Here's how the part is built. I have some questions about the finished solid (model axes, mm). Face numbers are marked on the shaded views. Coordinates: 2 decimals unless noted, no trailing zeros. Write each loop counter-clockwise with the first axis right and the second up, starting at its lowest first coordinate (ties: lowest second). Pieces come first, ordered by that corner, then holes. Notation, with made-up numbers: (55.5, 11) -> (69.5, 11) arc R22 ccw to (69.5, 25) -> close; hole circle Ø7 at (61.5, 42). An arc over 180 degrees is marked (long way). Use a Markdown table: item, result. Add a question column.
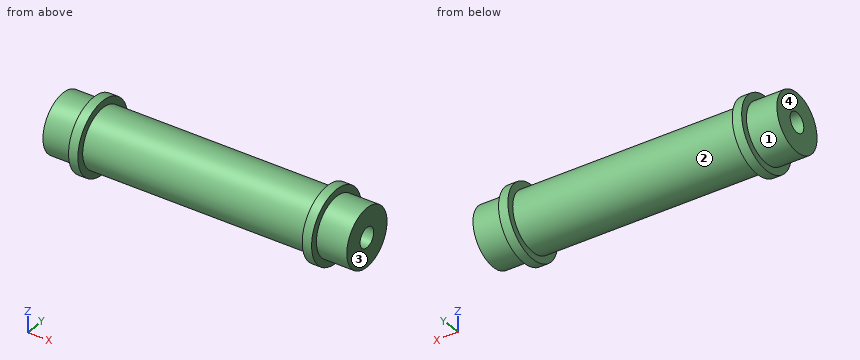
```python
from build123d import *

# Parameters (mm, degrees)
HOLE_WIZARD_M101_D     = 8.5
HOLE_WIZARD_M101_DEPTH = 22.5
HOLE_WIZARD_M101_TIP   = 2.553657631


with BuildPart() as part:
    # Эскиз1 → Повернуть1 (revolve)
    with BuildSketch(Plane.XY):
        Polygon((0, 0), (0, 12.5), (48, 12.5), (48, 15.5), (52, 15.5), (52, 12.5), (65, 12.5), (65, 0), align=None)
    revolve(axis=Axis((-1000, 0, 0), (1, 0, 0)))

    # Отверстие обработанное метчиком M101
    with Locations(Plane(origin=(65, 0, 0), x_dir=(0, 0, -1), z_dir=(1, 0, 0))):
        with Locations((0, 0)):
            Hole(HOLE_WIZARD_M101_D / 2, depth=HOLE_WIZARD_M101_DEPTH)
            with Locations((0, 0, -(HOLE_WIZARD_M101_DEPTH + HOLE_WIZARD_M101_TIP / 2))):  # 118° drill point
                Cone(0, HOLE_WIZARD_M101_D / 2, HOLE_WIZARD_M101_TIP, mode=Mode.SUBTRACT)

    # Зеркальное отражение1: part across plane


with BuildPart() as part_1:
    add(part.part)
    add(part.part.mirror(Plane(origin=(0, 0, 0), x_dir=(0, 0, 1), z_dir=(1, 0, 0))))


solid = part_1.part
```
Q1. Suppose I cut it at B-B, the plane x = -37.5. Write out the boundary of the cut face in (y, z), and give its area (3 significant figures).
Q2. Please list where these lines run through material, in increasing order: line 1 (Z direction, x = -51, y = 0); line 2 (X direction, y = 12, z = 8); line 3 (Z direction, x = 60, y = 0).
Q3. Suppose I cut it at D-D, the plane z = -6. Write out the boundary of the cut face in (x, y), and give its area (3 significant figures).
Q4. Thinking about a two-plate mould opening in X: for the marked faces 1, 2, 3 and 4, which applies, released by +X, released by -X, zero draft, split by the parting line, or undercut?
Q5. Suppose I cut it at C-C, the plane y = 7. Write out the boundary of the cut face in (x, z).
Q6. Will these pins go through, and if not, where does the flat tip stop? pin 1 (4 mm diameter, centred on x = 29.5, y = 9.5, fed in from +Z); pin 2 (1.5 mm diameter, centred on x = 40.5, y = 3, fed in from -Z); pin 3 (1 mm diameter, centred on x = -22.5, z = -5.5, fed in from +Y).
Q7. Suppose I cut it at A-A, the plane z = -14. Write out the boundary of the cut face in (x, y), and give its area (3 significant figures).
Answer key:
| question | item | result |
|---|---|---|
| 1 | outline | circle Ø25 at (0, 0) |
| 1 | area | 491 mm^2 |
| 2 | line 1 | z = -15.5 to -4.25, 4.25 to 15.5 |
| 2 | line 2 | x = -52 to -48, 48 to 52 |
| 2 | line 3 | z = -12.5 to -4.25, 4.25 to 12.5 |
| 3 | outline | (-65, -10.97) -> (-52, -10.97) -> (-52, -14.29) -> (-48, -14.29) -> (-48, -10.97) -> (48, -10.97) -> (48, -14.29) -> (52, -14.29) -> (52, -10.97) -> (65, -10.97) -> (65, 10.97) -> (52, 10.97) -> (52, 14.29) -> (48, 14.29) -> (48, 10.97) -> (-48, 10.97) -> (-48, 14.29) -> (-52, 14.29) -> (-52, 10.97) -> (-65, 10.97) -> close |
| 3 | area | 2,900 mm^2 |
| 4 | face 1 | zero draft |
| 4 | face 2 | undercut |
| 4 | face 3 | released by +X |
| 4 | face 4 | released by -X |
| 5 | outline | (-65, -10.36) -> (-52, -10.36) -> (-52, -13.83) -> (-48, -13.83) -> (-48, -10.36) -> (48, -10.36) -> (48, -13.83) -> (52, -13.83) -> (52, -10.36) -> (65, -10.36) -> (65, 10.36) -> (52, 10.36) -> (52, 13.83) -> (48, 13.83) -> (48, 10.36) -> (-48, 10.36) -> (-48, 13.83) -> (-52, 13.83) -> (-52, 10.36) -> (-65, 10.36) -> close |
| 6 | pin 1 | stops at z = 10 |
| 6 | pin 2 | stops at z = -12.3 |
| 6 | pin 3 | stops at y = 11.46 |
| 7 | outline | (-52, -6.65) -> (-48, -6.65) -> (-48, 6.65) -> (-52, 6.65) -> close; (48, -6.65) -> (52, -6.65) -> (52, 6.65) -> (48, 6.65) -> close |
| 7 | area | 106 mm^2 |
